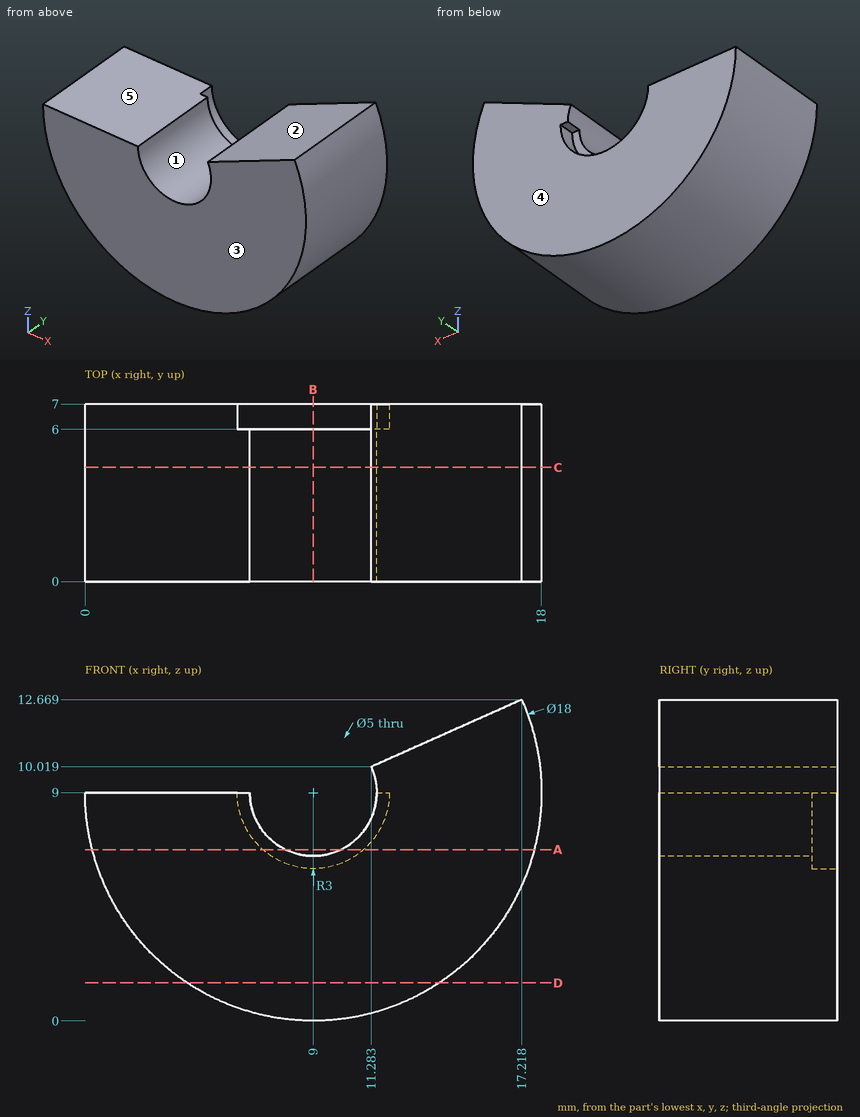
Geometry check sheet. Reference: drawing and pictorial views, mm from the part's lowest x, y, z. A direction names the side the tool comes from. Round coordinates to 2 decimals unless told otherwise and drop trailing zeros. Loops run counter-clockwise (first coordinate to the right, second up) from the corner with the lowest first, then second, coordinate; pieces in that order, holes last. Notation, with made-up numbers: (-8.75, -22.75) - (35.25, -22.75) arc R12 cw to (35.25, -11.75) - close; hole circle Ø7 at (15.25, 11). An arc over 180 degrees is marked (long way). Use a Markdown table: item, result.
Q1. Go/stop test with flat-tipped pins: P1, Ø0.9, axis at x = 9, z = 7.5, coming from the +Y side; P2, Ø1, axis at x = 2, y = 1, coming from the -Z side (1 decimal); P3, Ø2, axis at x = 14, y = 6, coming from the -Z side; P4, Ø3, axis at x = 3.5, y = 2, coming from the +Z side. Record where each tip stops, or that it passes through.
Solutions:
| item | result |
|---|---|
| P1 | passes through |
| P2 | stops at z = 2.8 |
| P3 | stops at z = 0.94 |
| P4 | stops at z = 9 |
Q2. Cross-section at C-C on y = 4.5. Record the cut outline in (x, z), plus the area to 3 significant figures.
Solutions:
| item | result |
|---|---|
| outline | (0, 9) arc R9 ccw (long way) to (17.22, 12.67) - (11.28, 10.02) arc R2.5 cw (long way) to (6.5, 9) - close |
| area | 133 mm2 |
Q3. Material ranges on line 1 (Z direction, x = 9, y = 3.5); line 2 (Z direction, x = 17, y = 1.5) (1 decimal); line 3 (X direction, y = 1, z = 1.5) (1 decimal), recorded low to high.
Solutions:
| item | result |
|---|---|
| line 1 | z = 0 to 6.5 |
| line 2 | z = 4.9 to 12.6 |
| line 3 | x = 4 to 14 |
Q4. Cross-section at D-D on z = 1.5. Record the cut outline in (x, y) (1 decimal).
Solutions:
| item | result |
|---|---|
| outline | (4, 0) - (14, 0) - (14, 7) - (4, 7) - close |
Q5. Cross-section at A-A on z = 6.75. Record the cut outline in (x, y).
Solutions:
| item | result |
|---|---|
| outline | (0.29, 0) - (7.91, 0) - (7.91, 6) - (7.02, 6) - (7.02, 7) - (0.29, 7) - close; (10.09, 0) - (17.71, 0) - (17.71, 7) - (10.98, 7) - (10.98, 6) - (10.09, 6) - close |
Q6. Access from +Z, -Z, +X, -X, +Y, -Y to the whole of each face (thin tool, end or side, straight path). Record for the marked faces 4 and 5.
Solutions:
| item | result |
|---|---|
| face 4 | +Z, -Z, +X, -X, +Y |
| face 5 | +Z, -X, +Y, -Y |
Q7. Cross-section at B-B on x = 9. Record the cut outline in (y, z).
Solutions:
| item | result |
|---|---|
| outline | (0, 0) - (7, 0) - (7, 6) - (6, 6) - (6, 6.5) - (0, 6.5) - close |
Q8. Draft check along Z on the marked faces 1, 2 and 3. Enter one of: released by +Z, released by -Z, zero draft, split by the parting line, or undercut.
Solutions:
| item | result |
|---|---|
| face 1 | undercut |
| face 2 | released by +Z |
| face 3 | zero draft |
